Job drawing, mm, ordinate dimensions from the low corner. One solid piece. Coordinates: 2 decimals unless noted, no trailing zeros. Loops run counter-clockwise (first coordinate to the right, second up) from the corner with the lowest first, then second, coordinate; pieces in that order, holes last. Notation, with made-up numbers: (-30.5, 55) - (-5.5, 55) arc R23 cw to (-5.5, 68) - close; hole circle Ø9 at (-17, -34.75). An arc over 180 degrees is marked (long way). Use a Markdown table: item, result. Add a question column.
1. Band-saw the part on A-A, the plane x = 45. Give the cut face in (y, z).
2. Wall check: probe 1 along Y at (x, z) = (45, 1.75); probe 2 along Y at (x, z) = (45, 11.5); probe 3 along Z at (x, y) = (68.5, 47.5). Give the ranges that are in metal, low to high. Write a range as [from, to].
3. Drop flat-ended pins along their axis: pin 1 (6 mm diameter, centred on y = 58.5, z = 10.5, fed in from -X); pin 2 (2 mm diameter, centred on y = 29.5, z = 3.5, fed in from -X); pin 3 (1 mm diameter, centred on y = 17, z = 3, fed in from +X). Give the stop position or say it passes through.
4. Band-saw the part on C-C, the plane z = 12.75. Give the cut face in (x, y), plus the area to 3 significant figures.
5. Pull direction X, two halves, no side cores. Call the marked faces 1, 2 and 3: pulls with the +X half, pulls with the -X half, needs draft (parallel to the pull), parting line crosses it, or undercut.
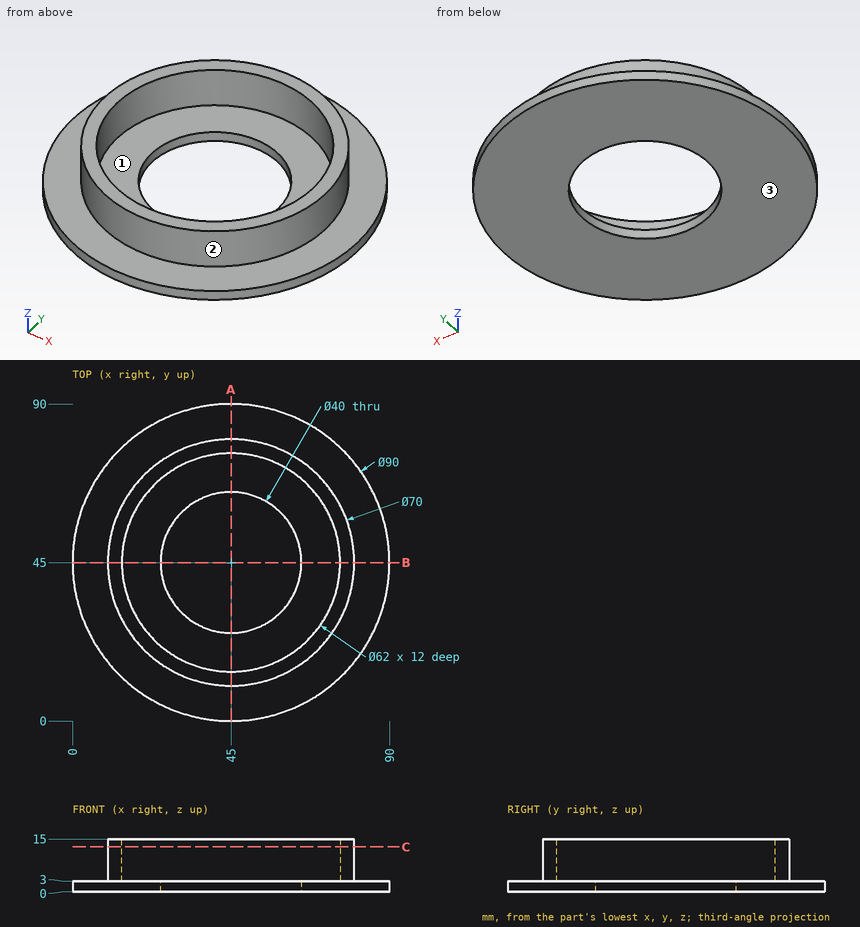
Geometry check:
| question | item | result |
|---|---|---|
| 1 | outline | (0, 0) - (25, 0) - (25, 3) - (14, 3) - (14, 15) - (10, 15) - (10, 3) - (0, 3) - close; (65, 0) - (90, 0) - (90, 3) - (80, 3) - (80, 15) - (76, 15) - (76, 3) - (65, 3) - close |
| 2 | probe 1 | y = [0, 25], [65, 90] |
| 2 | probe 2 | y = [10, 14], [76, 80] |
| 2 | probe 3 | z = [0, 3] |
| 3 | pin 1 | stops at x = 11.61 |
| 3 | pin 2 | stops at x = 2.45 |
| 3 | pin 3 | stops at x = 80.62 |
| 4 | outline | circle Ø70 at (45, 45); hole circle Ø62 at (45, 45) |
| 4 | area | 829 mm^2 |
| 5 | face 1 | undercut |
| 5 | face 2 | parting line crosses it |
| 5 | face 3 | needs draft |
